```python
from build123d import *

# Parameters (mm, degrees)
F1_DEPTH = 25
F0_R     = 2
F2_DEPTH = 3
F3_DEPTH = 5
F4_W     = 55
F4_H     = 4
F5_DEPTH = 85.001
F6_DEPTH = 6


with BuildPart() as f1:
    # F0 (on Top) → F1 (new body)
    with BuildSketch(Plane.XY):
        Polygon((-42.5, 0), (-22.5, 0), (22.5, 0), (42.5, 0), (42.5, 70), (22.5, 70), (22.5, 20), (0, 20), (-22.5, 20), (-22.5, 70), (-42.5, 70), align=None)
    extrude(amount=F1_DEPTH)

    # F0 (on Top) → F2 (join)
    with BuildSketch(Plane.XY):
        with BuildLine():
            ThreePointArc((-22.5, -70), (-30, -35), (-22.5, 0))
            Line((-22.5, 0), (-42.5, 0))
            Line((-42.5, 0), (-42.5, -70))
            Line((-42.5, -70), (-22.5, -70))
        make_face()
        with Locations((-32.5, -60)):
            Circle(F0_R, mode=Mode.SUBTRACT)
        with Locations((-32.5, -10)):
            Circle(F0_R, mode=Mode.SUBTRACT)
        with BuildLine():
            Line((42.5, 0), (22.5, 0))
            ThreePointArc((22.5, 0), (30, -35), (22.5, -70))
            Line((22.5, -70), (42.5, -70))
            Line((42.5, -70), (42.5, 0))
        make_face()
        with Locations((32.5, -60)):
            Circle(F0_R, mode=Mode.SUBTRACT)
        with Locations((32.5, -10)):
            Circle(F0_R, mode=Mode.SUBTRACT)
    extrude(amount=F2_DEPTH)

    # F0 (on Top) → F3 (join)
    with BuildSketch(Plane.XY):
        with Locations((-32.5, -10)):
            Circle(F0_R)
        with Locations((32.5, -10)):
            Circle(F0_R)
    extrude(amount=F3_DEPTH)

    # F4 (on face) → F5 (cut, through all)
    with BuildSketch(Plane(origin=(-42.5, 0, 0), x_dir=(0, -1, 0), z_dir=(-1, 0, 0))):
        Polygon((-15, 21), (-70, 21), (-70, 4), (-3, 4), (-3, 21), align=None)
        with Locations((-42.5, 23)):
            Rectangle(F4_W, F4_H)
    extrude(amount=-F5_DEPTH, mode=Mode.SUBTRACT)

    # F0 (on Top) → F6 (join)
    with BuildSketch(Plane.XY):
        with Locations((-32.5, -60)):
            Circle(F0_R)
        with Locations((32.5, -60)):
            Circle(F0_R)
    extrude(amount=F6_DEPTH)


solid = f1.part
```
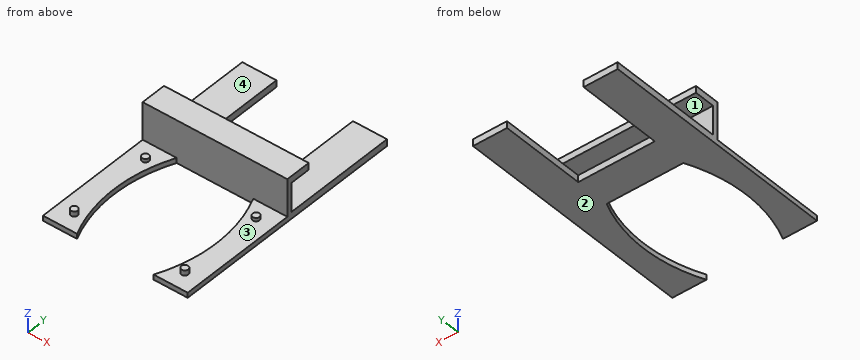
Can you work these out from the model? Positions are in its coordinate system, mm. Face numbers are marked on the shaded views. Give positions to 0.01 mm unless a question says otherwise; leave off trailing zeros. Order: outer loops, then holes, each group sorted by start corner. A loop starts at its lowest first (then second) coordinate and runs counter-clockwise, first axis right, second up. Notation, with made-up numbers: M 22,57.5 L 45,57.5 A21 cw 45,89.5 Z; hole C 62.5,-33.5 d6. An arc over 180 degrees is marked long. Write item = value, one per line. Start each with the question number.
Q1. Suppose I cut it at C-C (z = 1.5). Write out the boundary of the cut face in (x, y).
Q2. Suppose I cut it at D-D (y = 7). Write out the boundary of the cut face in (x, z).
Q3. We'd pull the mould along Z, two halves only. Please class the marked faces 1, 2, 3 and 4: pulls with the +Z half, pulls with the -Z half, needs draft (parallel to the pull), parting line crosses it, or undercut.
Q4. Will these pins go through, and if not, where does the flat tip stop? pin 1 Ø2 at (x, z) = (-7.5, 1) entering from +Y; pin 2 Ø3 at (x, y) = (32, -59) entering from +Z; pin 3 Ø8 at (x, z) = (26, 11) entering from -Y; pin 4 Ø6 at (x, y) = (-11, 6) entering from -Z.
Q5. Suppose I cut it at B-B (x = -3.5). Write out the boundary of the cut face in (y, z).
Q6. Suppose I cut it at A-A (y = 28.5). Write out the boundary of the cut face in (x, z).
Q7. I need wall thicknesses on probe 1 along Y at (x, z) = (-31, 14); probe 2 along Z at (x, y) = (24, 18). Which ranges of each line are inside material? Lowest first, please. Write a range as [from, to].
Check result:
q1.outline = M -42.5,-70 L -22.5,-70 A85.42 cw -22.5,0 L 22.5,0 A85.42 cw 22.5,-70 L 42.5,-70 L 42.5,70 L 22.5,70 L 22.5,20 L -22.5,20 L -22.5,70 L -42.5,70 Z
q2.outline = M -42.5,0 L 42.5,0 L 42.5,4 L -42.5,4 Z; M -42.5,21 L 42.5,21 L 42.5,25 L -42.5,25 Z
q3.face_1 = undercut
q3.face_2 = pulls with the -Z half
q3.face_3 = pulls with the +Z half
q3.face_4 = undercut
q4.pin_1 = 20
q4.pin_2 = 6
q4.pin_3 = 0
q4.pin_4 = 0
q5.outline = M 0,0 L 20,0 L 20,4 L 3,4 L 3,21 L 15,21 L 15,25 L 0,25 Z
q6.outline = M -42.5,0 L -22.5,0 L -22.5,4 L -42.5,4 Z; M 22.5,0 L 42.5,0 L 42.5,4 L 22.5,4 Z
q7.probe_1 = [0, 3]
q7.probe_2 = [0, 4]
